from build123d import *

# Parameters (mm, degrees)
SKETCH_1_W           = 21
SKETCH_1_H           = 21
EXTRUDE_1_DEPTH      = 60
EXTRUDE_1_DEPTH_BACK = 60
CUT_EXTRUDE_1_DEPTH  = 26


with BuildPart() as part:
    # Sketch 1 → Extrude 1 (new body, two sides)
    with BuildSketch(Plane.XY) as extrude_1_sk:
        with BuildLine():
            Line((-12.5, -12.5), (12.5, -12.5))
            Line((12.5, -12.5), (12.5, 11.5))
            ThreePointArc((12.5, 11.5), (12.207106781, 12.207106781), (11.5, 12.5))
            Line((11.5, 12.5), (-11.5, 12.5))
            ThreePointArc((-11.5, 12.5), (-12.207106781, 12.207106781), (-12.5, 11.5))
            Line((-12.5, 11.5), (-12.5, -12.5))
        make_face()
        Rectangle(SKETCH_1_W, SKETCH_1_H, mode=Mode.SUBTRACT)
    extrude(amount=EXTRUDE_1_DEPTH)
    extrude(extrude_1_sk.sketch, amount=-EXTRUDE_1_DEPTH_BACK)

    # Sketch 2 → Cut-Extrude 1 (cut, through all)
    with BuildSketch(Plane(origin=(12.5, 0, 0), x_dir=(0, 0, -1), z_dir=(1, 0, 0))):
        with BuildLine():
            Line((-232.745226472, -146.030996161), (-46.636895265, -12.5))
            ThreePointArc((-46.636895265, -12.5), (0, 2.5), (46.636895265, -12.5))
            Line((46.636895265, -12.5), (232.745226472, -146.030996161))
            Line((232.745226472, -146.030996161), (232.745226472, -604.143811438))
            Line((232.745226472, -604.143811438), (-232.745226472, -604.143811438))
            Line((-232.745226472, -604.143811438), (-232.745226472, -146.030996161))
        make_face()
    extrude(amount=-CUT_EXTRUDE_1_DEPTH, mode=Mode.SUBTRACT)


solid = part.part
Design review of the part built by this model. Coordinates are the model's own, in mm. A direction names the side the tool comes from. Round coordinates to 2 decimals unless told otherwise and drop trailing zeros. Write each loop counter-clockwise with the first axis right and the second up, starting at its lowest first coordinate (ties: lowest second). Pieces come first, ordered by that corner, then holes.
Item 1: Draft analysis for pull direction X (two halves, no side actions). For faces 3 (the flat face through (-12.5, 5, 1)), 4 (the flat face through (0, 10.5, 1)), 5 (the flat face through (0, -12.5, -53)), state which applies: released by +X, released by -X, zero draft, split by the parting line, or undercut.
Item 2: Consider section B-B on x = -6. Give the boundary of the cut face in (y, z).
Item 3: For faces 1 (the flat face through (-10.5, 5, 1)), 2 (the flat face through (0, -12.5, 53)), list the 3-axis set-ups (+Z, -Z, +X, -X, +Y, -Y) from which the entire face can be reached by the end or side of a thin tool; tool diameter is ignored.
Item 4: Consider section C-C on z = -50.5. Give the boundary of the cut face in (x, y), and give its area (3 significant figures).
Item 5: Consider section A-A on y = 4.5. Give the boundary of the cut face in (x, z).
Item 6: Consider section D-D on y = -0.5. Give the boundary of the cut face in (x, z), and give its area (3 significant figures).
Item 7: Wall thickness on L1, parallel to X at y = 7.5, z = -44; L2, parallel to Y at x = -6.75, z = -39: over which ranges is each line inside the solid? List them lowest first.
Item 8: For pin 1 Ø2 at (x, z) = (-7, -2.5) entering from -Y; pin 2 Ø12 at (x, z) = (-6.5, 37.5) entering from -Y, all flat-tipped, find the tip position at first contact; note any pin that passes through.
Check values:
1. face 3: released by -X
1. face 4: undercut
1. face 5: zero draft
2. outline: (-12.5, -60) - (-10.5, -60) - (-10.5, -43.71) arc R80 cw to (-12.5, -46.64) - close; (-12.5, 46.64) arc R80 cw to (-10.5, 43.71) - (-10.5, 60) - (-12.5, 60) - close; (10.5, -60) - (12.5, -60) - (12.5, 60) - (10.5, 60) - close
3. face 1: +Z, -Z
3. face 2: +Z, -Z, +X, -X, -Y
4. outline: (-12.5, -12.5) - (12.5, -12.5) - (12.5, 11.5) arc R1 ccw to (11.5, 12.5) - (-11.5, 12.5) arc R1 ccw to (-12.5, 11.5) - close; hole (-10.5, -10.5) - (10.5, -10.5) - (10.5, 10.5) - (-10.5, 10.5) - close
4. area: 184 mm2
5. outline: (-12.5, -60) - (-10.5, -60) - (-10.5, 60) - (-12.5, 60) - close; (10.5, -60) - (12.5, -60) - (12.5, 60) - (10.5, 60) - close
6. outline: (-12.5, -60) - (-10.5, -60) - (-10.5, -21.7) - (-12.5, -21.7) - close; (-12.5, 21.7) - (-10.5, 21.7) - (-10.5, 60) - (-12.5, 60) - close; (10.5, -60) - (12.5, -60) - (12.5, -21.7) - (10.5, -21.7) - close; (10.5, 21.7) - (12.5, 21.7) - (12.5, 60) - (10.5, 60) - close
6. area: 306 mm2
7. L1: x = -12.5 to -10.5, 10.5 to 12.5
7. L2: y = 10.5 to 12.5
8. pin 1: stops at y = 10.5
8. pin 2: stops at y = -9.39
